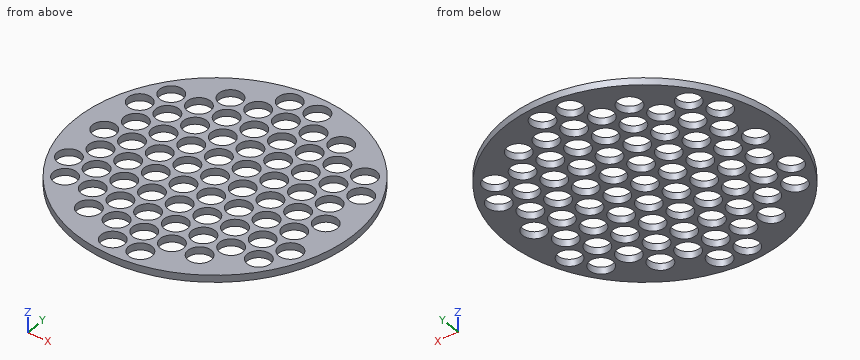
from build123d import *

# Parameters (mm, degrees)
F0_R     = 127
F0_R_2   = 10.668
F1_DEPTH = 6.35


with BuildPart() as f1:
    # F0 (on Top) → F1 (new body)
    with BuildSketch(Plane.XY):
        Circle(F0_R)
        with Locations((-88.9, -65.991136)):
            Circle(F0_R_2, mode=Mode.SUBTRACT)
        with Locations((-12.7, -109.985226)):
            Circle(F0_R_2, mode=Mode.SUBTRACT)
        with Locations((-50.8, -87.988181)):
            Circle(F0_R_2, mode=Mode.SUBTRACT)
        with Locations((-63.5, -65.991136)):
            Circle(F0_R_2, mode=Mode.SUBTRACT)
        with Locations((-38.1, -65.991136)):
            Circle(F0_R_2, mode=Mode.SUBTRACT)
        with Locations((-25.4, -87.988181)):
            Circle(F0_R_2, mode=Mode.SUBTRACT)
        with Locations((-12.7, -65.991136)):
            Circle(F0_R_2, mode=Mode.SUBTRACT)
        with Locations((-101.6, -43.994091)):
            Circle(F0_R_2, mode=Mode.SUBTRACT)
        with Locations((-76.2, -43.994091)):
            Circle(F0_R_2, mode=Mode.SUBTRACT)
        with Locations((-88.9, -21.997045)):
            Circle(F0_R_2, mode=Mode.SUBTRACT)
        with Locations((-50.8, -43.994091)):
            Circle(F0_R_2, mode=Mode.SUBTRACT)
        with Locations((-25.4, -43.994091)):
            Circle(F0_R_2, mode=Mode.SUBTRACT)
        with Locations((-63.5, -21.997045)):
            Circle(F0_R_2, mode=Mode.SUBTRACT)
        with Locations((-38.1, -21.997045)):
            Circle(F0_R_2, mode=Mode.SUBTRACT)
        with Locations((-12.7, -21.997045)):
            Circle(F0_R_2, mode=Mode.SUBTRACT)
        with Locations((12.7, -109.985226)):
            Circle(F0_R_2, mode=Mode.SUBTRACT)
        with Locations((0, -87.988181)):
            Circle(F0_R_2, mode=Mode.SUBTRACT)
        with Locations((25.4, -87.988181)):
            Circle(F0_R_2, mode=Mode.SUBTRACT)
        with Locations((12.7, -65.991136)):
            Circle(F0_R_2, mode=Mode.SUBTRACT)
        with Locations((50.8, -87.988181)):
            Circle(F0_R_2, mode=Mode.SUBTRACT)
        with Locations((38.1, -65.991136)):
            Circle(F0_R_2, mode=Mode.SUBTRACT)
        with Locations((63.5, -65.991136)):
            Circle(F0_R_2, mode=Mode.SUBTRACT)
        with Locations((88.9, -65.991136)):
            Circle(F0_R_2, mode=Mode.SUBTRACT)
        with Locations((0, -43.994091)):
            Circle(F0_R_2, mode=Mode.SUBTRACT)
        with Locations((25.4, -43.994091)):
            Circle(F0_R_2, mode=Mode.SUBTRACT)
        with Locations((50.8, -43.994091)):
            Circle(F0_R_2, mode=Mode.SUBTRACT)
        with Locations((12.7, -21.997045)):
            Circle(F0_R_2, mode=Mode.SUBTRACT)
        with Locations((38.1, -21.997045)):
            Circle(F0_R_2, mode=Mode.SUBTRACT)
        with Locations((76.2, -43.994091)):
            Circle(F0_R_2, mode=Mode.SUBTRACT)
        with Locations((101.6, -43.994091)):
            Circle(F0_R_2, mode=Mode.SUBTRACT)
        with Locations((63.5, -21.997045)):
            Circle(F0_R_2, mode=Mode.SUBTRACT)
        with Locations((88.9, -21.997045)):
            Circle(F0_R_2, mode=Mode.SUBTRACT)
        with Locations((-101.6, 0)):
            Circle(F0_R_2, mode=Mode.SUBTRACT)
        with Locations((-76.2, 0)):
            Circle(F0_R_2, mode=Mode.SUBTRACT)
        with Locations((-88.9, 21.997045)):
            Circle(F0_R_2, mode=Mode.SUBTRACT)
        with Locations((-101.6, 43.994091)):
            Circle(F0_R_2, mode=Mode.SUBTRACT)
        with Locations((-76.2, 43.994091)):
            Circle(F0_R_2, mode=Mode.SUBTRACT)
        with Locations((-50.8, 0)):
            Circle(F0_R_2, mode=Mode.SUBTRACT)
        with Locations((-63.5, 21.997045)):
            Circle(F0_R_2, mode=Mode.SUBTRACT)
        with Locations((-38.1, 21.997045)):
            Circle(F0_R_2, mode=Mode.SUBTRACT)
        with Locations((-25.4, 0)):
            Circle(F0_R_2, mode=Mode.SUBTRACT)
        with Locations((-12.7, 21.997045)):
            Circle(F0_R_2, mode=Mode.SUBTRACT)
        with Locations((-50.8, 43.994091)):
            Circle(F0_R_2, mode=Mode.SUBTRACT)
        with Locations((-25.4, 43.994091)):
            Circle(F0_R_2, mode=Mode.SUBTRACT)
        with Locations((-88.9, 65.991136)):
            Circle(F0_R_2, mode=Mode.SUBTRACT)
        with Locations((-63.5, 65.991136)):
            Circle(F0_R_2, mode=Mode.SUBTRACT)
        with Locations((-38.1, 65.991136)):
            Circle(F0_R_2, mode=Mode.SUBTRACT)
        with Locations((-50.8, 87.988181)):
            Circle(F0_R_2, mode=Mode.SUBTRACT)
        with Locations((-12.7, 65.991136)):
            Circle(F0_R_2, mode=Mode.SUBTRACT)
        with Locations((-25.4, 87.988181)):
            Circle(F0_R_2, mode=Mode.SUBTRACT)
        with Locations((-12.7, 109.985226)):
            Circle(F0_R_2, mode=Mode.SUBTRACT)
        Circle(F0_R_2, mode=Mode.SUBTRACT)
        with Locations((25.4, 0)):
            Circle(F0_R_2, mode=Mode.SUBTRACT)
        with Locations((12.7, 21.997045)):
            Circle(F0_R_2, mode=Mode.SUBTRACT)
        with Locations((50.8, 0)):
            Circle(F0_R_2, mode=Mode.SUBTRACT)
        with Locations((38.1, 21.997045)):
            Circle(F0_R_2, mode=Mode.SUBTRACT)
        with Locations((0, 43.994091)):
            Circle(F0_R_2, mode=Mode.SUBTRACT)
        with Locations((25.4, 43.994091)):
            Circle(F0_R_2, mode=Mode.SUBTRACT)
        with Locations((50.8, 43.994091)):
            Circle(F0_R_2, mode=Mode.SUBTRACT)
        with Locations((76.2, 0)):
            Circle(F0_R_2, mode=Mode.SUBTRACT)
        with Locations((63.5, 21.997045)):
            Circle(F0_R_2, mode=Mode.SUBTRACT)
        with Locations((88.9, 21.997045)):
            Circle(F0_R_2, mode=Mode.SUBTRACT)
        with Locations((101.6, 0)):
            Circle(F0_R_2, mode=Mode.SUBTRACT)
        with Locations((76.2, 43.994091)):
            Circle(F0_R_2, mode=Mode.SUBTRACT)
        with Locations((101.6, 43.994091)):
            Circle(F0_R_2, mode=Mode.SUBTRACT)
        with Locations((12.7, 65.991136)):
            Circle(F0_R_2, mode=Mode.SUBTRACT)
        with Locations((0, 87.988181)):
            Circle(F0_R_2, mode=Mode.SUBTRACT)
        with Locations((25.4, 87.988181)):
            Circle(F0_R_2, mode=Mode.SUBTRACT)
        with Locations((38.1, 65.991136)):
            Circle(F0_R_2, mode=Mode.SUBTRACT)
        with Locations((50.8, 87.988181)):
            Circle(F0_R_2, mode=Mode.SUBTRACT)
        with Locations((12.7, 109.985226)):
            Circle(F0_R_2, mode=Mode.SUBTRACT)
        with Locations((63.5, 65.991136)):
            Circle(F0_R_2, mode=Mode.SUBTRACT)
        with Locations((88.9, 65.991136)):
            Circle(F0_R_2, mode=Mode.SUBTRACT)
    extrude(amount=F1_DEPTH)


solid = f1.part
Build history of the part. All positions in model axes, mm. Round coordinates to 2 decimals unless told otherwise and drop trailing zeros. Loops run counter-clockwise (first coordinate to the right, second up) from the corner with the lowest first, then second, coordinate; pieces in that order, holes last. Notation, with made-up numbers: (-12.75, 18) -> (24.25, 18) arc R13 ccw to (24.25, 40) -> close; hole circle Ø1 at (18.25, 4.5). An arc over 180 degrees is marked (long way). Use CSV: the item, a comma, the result in double quotes. Start each with the question number.
Q1. Drill centre lines: L1, parallel to Y at x = -0.5, z = 5.5; L2, parallel to Y at x = 88.9, z = 4.5; L3, parallel to X at y = -92, z = 0.5. Where is each one in solid material? Low to high.
Q2. Saw through at B-B on z = 1. Count the separate pieces of the cut face and the enclosed holes in it, and give its area (3 significant figures).
Q3. Saw through at A-A on y = -95. Give the cut face in (x, z), and give its area (3 significant figures).
Q4. Flat gauge pins, fed straight in: pin 1 Ø1 at (y, z) = (-74.5, 1) entering from -X; pin 2 Ø3 at (y, z) = (23, 2.5) entering from -X; pin 3 Ø1 at (x, z) = (-88, 1) entering from +Y. Where does each tip first touch, or does it go through?
Solutions:
1,L1,"y = -127 to -98.64, -77.33 to -54.65, -33.34 to -10.66, 10.66 to 33.34, 54.65 to 77.33, 98.64 to 127"
1,L2,"y = -90.7 to -76.66, -55.32 to -32.67, -11.33 to 11.33, 32.67 to 55.32, 76.66 to 90.7"
1,L3,"x = -87.55 to -60.68, -40.92 to -35.28, -15.52 to -9.88, 9.88 to 15.52, 35.28 to 40.92, 60.68 to 87.55"
2,separate pieces,"1"
2,enclosed holes,"73"
2,area,"24,600 mm^2"
3,outline,"(-84.29, 0) -> (-58.84, 0) -> (-58.84, 6.35) -> (-84.29, 6.35) -> close; (-42.76, 0) -> (-33.44, 0) -> (-33.44, 6.35) -> (-42.76, 6.35) -> close; (-17.36, 0) -> (-8.04, 0) -> (-8.04, 6.35) -> (-17.36, 6.35) -> close; (8.04, 0) -> (17.36, 0) -> (17.36, 6.35) -> (8.04, 6.35) -> close; (33.44, 0) -> (42.76, 0) -> (42.76, 6.35) -> (33.44, 6.35) -> close; (58.84, 0) -> (84.29, 0) -> (84.29, 6.35) -> (58.84, 6.35) -> close"
3,area,"560 mm^2"
4,pin 1,"stops at x = -103.21"
4,pin 2,"stops at x = -125.17"
4,pin 3,"stops at y = 92.05"
